from build123d import *

# Parameters (mm, degrees)
SKETCH1_W               = 36
SKETCH1_H               = 16
BOSS_EXTRUDE1_DEPTH     = 3
SKETCH3_W               = 4
SKETCH3_H               = 16
BOSS_EXTRUDE2_DEPTH     = 16
BOSS_EXTRUDE3_DEPTH     = 3
CUT_EXTRUDE2_DEPTH      = 29.722813233
CUT_EXTRUDE2_DEPTH_BACK = 29.722813233
FILLET1_START           = -5
FILLET1_DEPTH           = 3
FILLET1_START_2         = 2
FILLET1_2_DEPTH         = 3
SKETCH7_R               = 5
CUT_EXTRUDE3_DEPTH      = 6
SKETCH8_R               = 1.5
CUT_EXTRUDE5_DEPTH      = 6
SKETCH12_W              = 36
SKETCH12_H              = 3
BOSS_EXTRUDE4_DEPTH     = 2
SKETCH13_W              = 36
SKETCH13_H              = 3
BOSS_EXTRUDE5_DEPTH     = 2
SKETCH14_W              = 20
SKETCH14_H              = 3
BOSS_EXTRUDE6_DEPTH     = 2
SKETCH15_W              = 20
SKETCH15_H              = 3
BOSS_EXTRUDE7_DEPTH     = 2
SKETCH16_W              = 20
SKETCH16_H              = 4
CUT_EXTRUDE6_DEPTH      = 6
CHAMFER1_SIZE           = 2
FILLET3_R               = 3


with BuildPart() as part:
    # Sketch1 → Boss-Extrude1 (new body)
    with BuildSketch(Plane(origin=(0, 0, 0), x_dir=(1, 0, 0), z_dir=(0, 1, 0))):
        Rectangle(SKETCH1_W, SKETCH1_H)
    extrude(amount=BOSS_EXTRUDE1_DEPTH)

    # Sketch3 → Boss-Extrude2 (add)
    with BuildSketch(Plane(origin=(0, 3, 0), x_dir=(1, 0, 0), z_dir=(0, 1, 0))):
        Rectangle(SKETCH3_W, SKETCH3_H)
    extrude(amount=BOSS_EXTRUDE2_DEPTH)

    # Sketch4 → Boss-Extrude3 (add)
    with BuildSketch(Plane.ZY.offset(2)):
        with BuildLine():
            Line((-8, 3), (1.5e-08, 3))
            ThreePointArc((1.5e-08, 3), (-5.656854244, 5.343145745), (-8, 11))
            Line((-8, 11), (-8, 3))
        make_face()
    boss_extrude3 = extrude(amount=BOSS_EXTRUDE3_DEPTH)

    # Mirror1: Boss-Extrude3 across plane
    add(boss_extrude3.mirror(Plane(origin=(0, 0, 0), x_dir=(0, 0, 1), z_dir=(1, 0, 0))))

    # Sketch6 → Cut-Extrude2 (cut, two sides: drawn at the far end of the back side and taken through both)
    with BuildSketch(Plane.ZY.offset(2).offset(-CUT_EXTRUDE2_DEPTH_BACK)):
        with BuildLine():
            Line((-8, 19), (-8, 11))
            ThreePointArc((-8, 11), (-5.656854249, 16.656854249), (0, 19))
            Line((0, 19), (-8, 19))
        make_face()
        with BuildLine():
            ThreePointArc((0, 19), (5.656854249, 16.656854249), (8, 11))
            Line((8, 11), (8, 19))
            Line((8, 19), (0, 19))
        make_face()
    extrude(amount=CUT_EXTRUDE2_DEPTH + CUT_EXTRUDE2_DEPTH_BACK, mode=Mode.SUBTRACT)

    # Fillet1: read off the stored shape, not the designer's step
    # Fillet1 outline → Fillet1 (cut)
    with BuildSketch(Plane.YZ.offset(FILLET1_START)):
        with BuildLine():
            ThreePointArc((11, -8), (8.333333334, -7.542472332), (5.971685112, -6.222222222))
            ThreePointArc((5.971685112, -6.222222222), (6.285954792, -7.333333333), (5.343145751, -8))
            Line((5.343145751, -8), (11, -8))
        make_face()
    extrude(amount=FILLET1_DEPTH, mode=Mode.SUBTRACT)

    # Fillet1 2 outline → Fillet1 2 (cut)
    with BuildSketch(Plane.YZ.offset(FILLET1_START_2)):
        with BuildLine():
            ThreePointArc((11, -8), (8.333333334, -7.542472332), (5.971685112, -6.222222222))
            ThreePointArc((5.971685112, -6.222222222), (6.285954792, -7.333333333), (5.343145751, -8))
            Line((5.343145751, -8), (11, -8))
        make_face()
    extrude(amount=FILLET1_2_DEPTH, mode=Mode.SUBTRACT)

    # Sketch7 → Cut-Extrude3 (cut)
    with BuildSketch(Plane.ZY.offset(2)):
        with Locations((0, 11)):
            Circle(SKETCH7_R)
    extrude(amount=-CUT_EXTRUDE3_DEPTH, mode=Mode.SUBTRACT)

    # Sketch8 → Cut-Extrude5 (cut)
    with BuildSketch(Plane(origin=(0, 3, 0), x_dir=(1, 0, 0), z_dir=(0, 1, 0))):
        with Locations(Location((-14.85, 4.95, 0), (0, 0, 270))):
            Circle(SKETCH8_R)
        with Locations(Location((14.85, 4.95, 0), (0, 0, 90))):
            Circle(SKETCH8_R)
        with Locations(Location((14.85, -4.95, 0), (0, 0, 270))):
            Circle(SKETCH8_R)
        with Locations(Location((-14.85, -4.95, 0), (0, 0, 90))):
            Circle(SKETCH8_R)
    extrude(amount=-CUT_EXTRUDE5_DEPTH, mode=Mode.SUBTRACT)

    # Sketch12 → Boss-Extrude4 (add)
    with BuildSketch(Plane.XY.offset(8)):
        with Locations((0, 1.5)):
            Rectangle(SKETCH12_W, SKETCH12_H)
    extrude(amount=BOSS_EXTRUDE4_DEPTH)

    # Sketch13 → Boss-Extrude5 (add)
    with BuildSketch(Plane(origin=(0, 0, -8), x_dir=(-1, 0, 0), z_dir=(0, 0, -1))):
        with Locations((0, 1.5)):
            Rectangle(SKETCH13_W, SKETCH13_H)
    extrude(amount=BOSS_EXTRUDE5_DEPTH)

    # Sketch14 → Boss-Extrude6 (add)
    with BuildSketch(Plane.ZY.offset(18)):
        with Locations((0, 1.5)):
            Rectangle(SKETCH14_W, SKETCH14_H)
    extrude(amount=BOSS_EXTRUDE6_DEPTH)

    # Sketch15 → Boss-Extrude7 (add)
    with BuildSketch(Plane(origin=(18, 0, 0), x_dir=(0, 0, -1), z_dir=(1, 0, 0))):
        with Locations((0, 1.5)):
            Rectangle(SKETCH15_W, SKETCH15_H)
    extrude(amount=BOSS_EXTRUDE7_DEPTH)

    # Sketch16 → Cut-Extrude6 (cut)
    with BuildSketch(Plane(origin=(0, 3, 0), x_dir=(1, 0, 0), z_dir=(0, 1, 0))):
        with Locations((0, -10)):
            Rectangle(SKETCH16_W, SKETCH16_H)
    extrude(amount=-CUT_EXTRUDE6_DEPTH, mode=Mode.SUBTRACT)

    # Chamfer1
    chamfer1_edges = [part.edges().sort_by_distance(p)[0] for p in [
        (6, 3, 8),
        (-6, 3, 8),
    ]]
    chamfer(chamfer1_edges, length=CHAMFER1_SIZE)

    # Fillet3
    fillet3_edges = [part.edges().sort_by_distance(p)[0] for p in [
        (-20, 1.5, -10),
        (-20, 1.5, 10),
        (20, 1.5, 10),
        (20, 1.5, -10),
        (-10, 1.5, 10),
    ]]
    fillet(fillet3_edges, radius=FILLET3_R)


solid = part.part
Geometry: final body of the model. Coordinates: model frame, mm. A direction names the side the tool comes from. Coordinates: 2 decimals unless noted, no trailing zeros. Order: outer loops, then holes, each group sorted by start corner. A loop starts at its lowest first (then second) coordinate and runs counter-clockwise, first axis right, second up.
1) Section D-D (z = 8.5). Return loops of the section in (x, y), then the cut area to 3 significant figures.
Result sheet:
outline: (-19.6, 0) - (-10.4, 0) - (-10.4, 3) - (-19.6, 3) - close; (10, 0) - (19.6, 0) - (19.6, 3) - (10, 3) - close
area: 56.4 mm2
2) Draft query along Z for faces 6 (the flat face through (0, 6, -8)), 7 (the flat face through (5, 4, -6)), 8 (the cylindrical face through (-0.028, 15.957, -0.651)). Return one class per face: released by +Z, released by -Z, zero draft, split by the parting line, or undercut.
Result sheet:
face 6: released by -Z
face 7: zero draft
face 8: undercut
3) Set-up query: faces 1 (the cylindrical face through (3.48, 6.29, -7.32)), 2 (the flat face through (-10, 2.62, 6.62)), 3 (the cylindrical face through (-3.48, 3.76, -3.4)), 4 (the flat face through (-5, 4, -6)), 5 (the cylindrical face through (-3.52, 6.29, -7.32)). Return all of +Z, -Z, +X, -X, +Y, -Y with unobstructed straight access to the full face (end or side cutting, diameter ignored); none if empty.
Result sheet:
face 1: +X, +Y
face 2: +Z, +Y
face 3: +Z, -X, +Y
face 4: +Z, -Z, -X, +Y
face 5: -X, +Y
4) Ray query, probe 1 along X at (y, z) = (1, -4.95); probe 2 along Y at (x, z) = (-14, 9.25); probe 3 along X at (y, z) = (2, -3.75). Return the intervals inside material, ascending.
Result sheet:
probe 1: x = -20 to -16.35, -13.35 to 13.35, 16.35 to 20
probe 2: y = 0 to 3
probe 3: x = -20 to -15.75, -13.95 to 13.95, 15.75 to 20
5) Section C-C (x = 1). Return loops of the section in (y, z), then the cut area to 3 significant figures.
Result sheet:
outline: (0, -10) - (3, -10) - (3, -8) - (11, -8) arc R8 ccw to (11, 8) - (0, 8) - close; hole circle Ø10 at (11, 0)
area: 204 mm2
6) Section A-A (x = -14.85). Return loops of the section in (y, z).
Result sheet:
outline: (0, -10) - (3, -10) - (3, -6.45) - (0, -6.45) - close; (0, -3.45) - (3, -3.45) - (3, 3.45) - (0, 3.45) - close; (0, 6.45) - (3, 6.45) - (3, 10) - (0, 10) - close
7) Section B-B (y = 15). Return loops of the section in (x, z), then the cut area to 3 significant figures.
Result sheet:
outline: (-2, -6.93) - (2, -6.93) - (2, -3) - (-2, -3) - close; (-2, 3) - (2, 3) - (2, 6.93) - (-2, 6.93) - close
area: 31.4 mm2
8) First-contact query: P1, Ø1.7, axis at y = 4.5, z = -3.5, coming from the +X side; P2, Ø1.8, axis at x = 14.85, z = 4.95, coming from the -Y side; P3, Ø3, axis at x = 8, z = 1, coming from the +Y side; P4, Ø4, axis at x = 1, y = 7, coming from the -Z side. Flat tips, straight axial feed; report the tip coordinate or a pass-through.
Result sheet:
P1: stops at x = 5
P2: passes through
P3: stops at y = 3
P4: stops at z = -8
